Answer from the drawing. Dimensions are ordinates in mm from the lowest x, y and z of the part. Round coordinates to 2 decimals unless told otherwise and drop trailing zeros. Write each loop counter-clockwise with the first axis right and the second up, starting at its lowest first coordinate (ties: lowest second). Pieces come first, ordered by that corner, then holes. Notation, with made-up numbers: (58, 40.5) - (110, 40.5) arc R24 ccw to (110, 66.5) - close; hole circle Ø8 at (79, 82). An arc over 180 degrees is marked (long way). Write item = value, one per line. Start each with the question number.
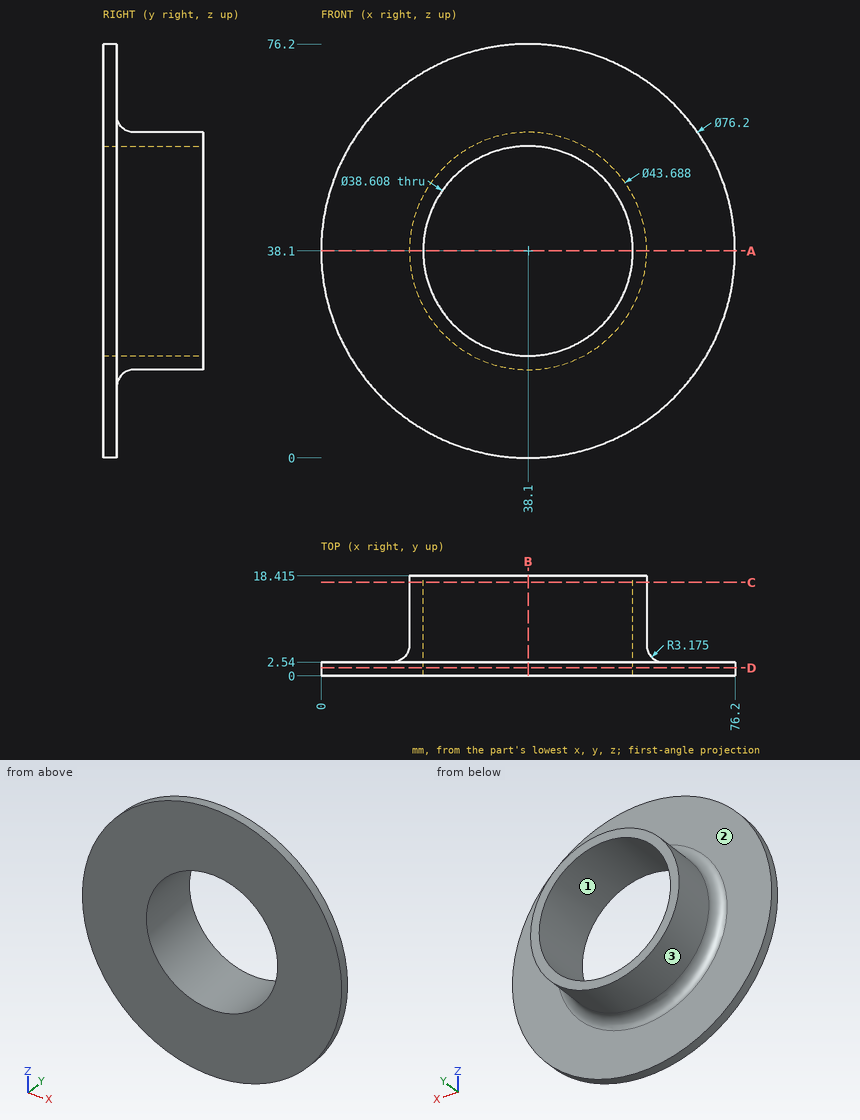
1. Find section C-C on y = 17.25. Give the vertices of the cut face in (x, z).
2. Find section A-A on z = 38.1. Give the vertices of the cut face in (x, y) (3 decimals), plus the area to 3 significant figures.
3. Find section D-D on y = 1.5. Give the vertices of the cut face in (x, z).
4. For a pull along X with two mould halves and no side action, classify the marked faces 1, 2 and 3 as released by +X, released by -X, zero draft, split by the parting line, or undercut.
5. Each of these flat-tipped pins is pushed along its axis until it touches: pin 1 (8 mm diameter, centred on x = 12.5, z = 26.5, fed in from +Y); pin 2 (10 mm diameter, centred on x = 49, y = 4, fed in from -Z); pin 3 (2 mm diameter, centred on y = 8.5, z = 59, fed in from +X). Where does it stop, or does it pass through?
6. Consider line 1 (Z direction, x = 38.1, y = 8.25); line 2 (Y direction, x = 22.5, z = 15); line 3 (X direction, y = 5.5, z = 40). Determine where each line is inside the solid, lowest interval first.
7. Find section B-B on x = 38.1. Give the vertices of the cut face in (y, z) (3 decimals).
Answer key:
q1.outline = circle Ø43.69 at (38.1, 38.1); hole circle Ø38.61 at (38.1, 38.1)
q2.outline = (0, 0) - (18.796, 0) - (18.796, 18.415) - (16.256, 18.415) - (16.256, 5.715) arc R3.175 cw to (13.081, 2.54) - (0, 2.54) - close; (57.404, 0) - (76.2, 0) - (76.2, 2.54) - (63.119, 2.54) arc R3.175 cw to (59.944, 5.715) - (59.944, 18.415) - (57.404, 18.415) - close
q2.area = 180 mm²
q3.outline = circle Ø76.2 at (38.1, 38.1); hole circle Ø38.61 at (38.1, 38.1)
q4.face_1 = undercut
q4.face_2 = zero draft
q4.face_3 = split by the parting line
q5.pin_1 = 2.67
q5.pin_2 = 0.49
q5.pin_3 = 47.11
q6.line_1 = 16.26 to 18.8, 57.4 to 59.94
q6.line_2 = 0 to 2.54
q6.line_3 = 16.33 to 18.89, 57.31 to 59.87
q7.outline = (0, 0) - (2.54, 0) - (2.54, 13.081) arc R3.175 cw to (5.715, 16.256) - (18.415, 16.256) - (18.415, 18.796) - (0, 18.796) - close; (0, 57.404) - (18.415, 57.404) - (18.415, 59.944) - (5.715, 59.944) arc R3.175 cw to (2.54, 63.119) - (2.54, 76.2) - (0, 76.2) - close
